Can you work these out from the model? Positions are in its coordinate system, mm. A direction names the side the tool comes from. Coordinates: 2 decimals unless noted, no trailing zeros. Loops run counter-clockwise (first coordinate to the right, second up) from the corner with the lowest first, then second, coordinate; pieces in that order, holes last. Notation, with made-up numbers: M -10,-23.75 L 35,-23.75 A14 cw 35,-14.75 Z; hole C 13.5,-10.75 d7. An arc over 180 degrees is marked long. Answer as a JSON object with one key per item and string values. Group by question number.
Item 1: Suppose I cut it at A-A (z = -30). Count the separate pieces of the cut face and the enclosed holes in it, then the cut area to 3 significant figures.
Item 2: Suppose I cut it at B-B (x = -3). Write out the boundary of the cut face in (y, z), then the cut area to 3 significant figures.
Item 3: If I drill on line 1 (Z direction, x = -74, y = 3.75); line 2 (Z direction, x = 70, y = 5.25); line 3 (X direction, y = 3.5, z = -10), over which ranges is the centre line in solid material (lowest first)?
Item 4: Which directions (+Z, -Z, +X, -X, +Y, -Y) give clear straight access to the entire face, cutting with the end or side of a thin tool? Please do faces 4 (the cylindrical face through (-97.15, 3.22, -41.99)), 5 (the flat face through (0, 3, -17.5)).
Item 5: We'd pull the mould along X, two halves only. Please class faces 1 (the cylindrical face through (-61.617, 3.131, 6.67)), 2 (the cylindrical face through (-97.15, 3.22, 41.99)), 3 (the cylindrical face through (96.99, 3.22, 42.15)): +X half, -X half, draft (parallel to the pull), parting line (faces both ways), or undercut.
Item 6: Suppose I cut it at C-C (z = -10). Write out the boundary of the cut face in (x, y), then the cut area to 3 significant figures.
Item 7: I'm going to push a flat-ended pin straight in: pin 1 Ø6 at (x, z) = (32.5, 30) entering from +Y. Where does the tip first touch, or does it pass through?
```python
from build123d import *

# Parameters (mm, degrees)
SKETCH1_W                                          = 200
SKETCH1_H                                          = 90
BOSS_EXTRUDE1_DEPTH                                = 6.35
CSK_FOR_10_FLAT_HEAD_MACHINE_SCREW_100_D           = 5.1054
CSK_FOR_10_FLAT_HEAD_MACHINE_SCREW_100_CSINK_D     = 9.779
CSK_FOR_10_FLAT_HEAD_MACHINE_SCREW_100_CSINK_ANGLE = 100
M4_CLEARANCE_HOLE1_D                               = 4.5
SKETCH9_W                                          = 35
SKETCH9_H                                          = 35
CUT_EXTRUDE1_DEPTH                                 = 6.35
FILLET1_R                                          = 10
FILLET2_R                                          = 5
F_8_32_TAPPED_HOLE1_D                              = 3.175
SKETCH15_R                                         = 1.75
CUT_EXTRUDE2_DEPTH                                 = 7.35


with BuildPart() as part:
    # Sketch1 → Boss-Extrude1 (new body)
    with BuildSketch(Plane(origin=(0, 0, 0), x_dir=(1, 0, 0), z_dir=(0, 1, 0))):
        Rectangle(SKETCH1_W, SKETCH1_H)
    extrude(amount=BOSS_EXTRUDE1_DEPTH)

    # CSK for #10 Flat Head Machine Screw (100)1 (through all)
    with Locations(Plane(origin=(0, 6.35, 0), x_dir=(1, 0, 0), z_dir=(0, 1, 0))):
        with Locations((-32.5, 30), (-32.5, -30), (32.5, -30), (32.5, 30)):
            CounterSinkHole(CSK_FOR_10_FLAT_HEAD_MACHINE_SCREW_100_D / 2, CSK_FOR_10_FLAT_HEAD_MACHINE_SCREW_100_CSINK_D / 2, counter_sink_angle=CSK_FOR_10_FLAT_HEAD_MACHINE_SCREW_100_CSINK_ANGLE)

    # M4 Clearance Hole1 (through all)
    with Locations(Plane(origin=(0, 6.35, 0), x_dir=(1, 0, 0), z_dir=(0, 1, 0))):
        with Locations((-90, -30), (-90, 30), (90, 30), (90, -30), (-70, -30), (-70, 30), (50, 30), (50, -30)):
            Hole(M4_CLEARANCE_HOLE1_D / 2)

    # Sketch9 → Cut-Extrude1 (cut)
    with BuildSketch(Plane(origin=(0, 6.35, 0), x_dir=(1, 0, 0), z_dir=(0, 1, 0))):
        Rectangle(SKETCH9_W, SKETCH9_H)
    extrude(amount=-CUT_EXTRUDE1_DEPTH, mode=Mode.SUBTRACT)

    # Fillet1
    fillet1_edges = [part.edges().sort_by_distance(p)[0] for p in [
        (100, 3.175, 45),
        (-100, 3.175, 45),
        (-100, 3.175, -45),
        (100, 3.175, -45),
    ]]
    fillet(fillet1_edges, radius=FILLET1_R)

    # Fillet2
    fillet2_edges = [part.edges().sort_by_distance(p)[0] for p in [
        (17.5, 3.175, -17.5),
        (17.5, 3.175, 17.5),
        (-17.5, 3.175, 17.5),
        (-17.5, 3.175, -17.5),
    ]]
    fillet(fillet2_edges, radius=FILLET2_R)

    # #8-32 Tapped Hole1 (through all)
    with Locations(Plane(origin=(0, 6.35, 0), x_dir=(1, 0, 0), z_dir=(0, 1, 0))):
        with Locations((70, 23.923457084), (70, -23.923457084)):
            Hole(F_8_32_TAPPED_HOLE1_D / 2)

    # Sketch15 → Cut-Extrude2 (cut, through all)
    with BuildSketch(Plane(origin=(0, 0, 0), x_dir=(-1, 0, 0), z_dir=(0, -1, 0))):
        with Locations((74, 6)):
            Circle(SKETCH15_R)
        with Locations((60, 6)):
            Circle(SKETCH15_R)
        with Locations((60, -6)):
            Circle(SKETCH15_R)
        with Locations((74, -6)):
            Circle(SKETCH15_R)
    extrude(amount=-CUT_EXTRUDE2_DEPTH, mode=Mode.SUBTRACT)


solid = part.part
```
From the geometry:
{
 "1": {"separate pieces": "7", "enclosed holes": "0", "area": "1,080 mm2"},
 "2": {"outline": "M 0,-45 L 6.35,-45 L 6.35,-17.5 L 0,-17.5 Z; M 0,17.5 L 6.35,17.5 L 6.35,45 L 0,45 Z", "area": "349 mm2"},
 "3": {"line 1": "-45 to -7.75, -4.25 to 4.25, 7.75 to 45", "line 2": "-45 to -25.51, -22.34 to 22.34, 25.51 to 45", "line 3": "-100 to -17.5, 17.5 to 100"},
 "4": {"face 4": "-Z, -X, +Y, -Y", "face 5": "+Y, -Y"},
 "5": {"face 1": "undercut", "face 2": "-X half", "face 3": "+X half"},
 "6": {"outline": "M -100,0 L -17.5,0 L -17.5,6.35 L -100,6.35 Z; M 17.5,0 L 100,0 L 100,6.35 L 17.5,6.35 Z", "area": "1,050 mm2"},
 "7": {"pin 1": "y = 4.76"}
}
